```python
from build123d import *

# Parameters (mm, degrees)
SKETCH1_R           = 11
SKETCH1_R_2         = 5.375
SKETCH1_R_3         = 1.475
BOSS_EXTRUDE1_DEPTH = 3
SKETCH6_R           = 1.475
CUT_EXTRUDE1_DEPTH  = 11


with BuildPart() as part:
    # Sketch1 → Boss-Extrude1 (new body)
    with BuildSketch(Plane(origin=(0, 0, 0), x_dir=(1, 0, 0), z_dir=(0, 1, 0))):
        with Locations(Location((0, 0, 0), (0, 0, 270))):
            Circle(SKETCH1_R)
        with Locations(Location((0, 0, 0), (0, 0, 270))):
            Circle(SKETCH1_R_2, mode=Mode.SUBTRACT)
        with Locations(Location((-5.657708628, -5.655999742, 0), (0, 0, 270))):
            Circle(SKETCH1_R_3, mode=Mode.SUBTRACT)
        with Locations(Location((-5.657708628, 5.655999742, 0), (0, 0, 270))):
            Circle(SKETCH1_R_3, mode=Mode.SUBTRACT)
        with Locations(Location((5.657708628, 5.655999742, 0), (0, 0, 270))):
            Circle(SKETCH1_R_3, mode=Mode.SUBTRACT)
        with Locations(Location((5.657708628, -5.655999742, 0), (0, 0, 270))):
            Circle(SKETCH1_R_3, mode=Mode.SUBTRACT)
    extrude(amount=BOSS_EXTRUDE1_DEPTH)

    # Sketch5 → Revolve1 (revolve)
    with BuildSketch(Plane(origin=(0, 0, 0), x_dir=(0, 0, -1), z_dir=(1, 0, 0))):
        Polygon((5.375, 4.5), (5.375, 3), (11, 3), align=None)
    revolve(axis=Axis((0, 0, 0), (0, 1, 0)))

    # Sketch6 → Cut-Extrude1 (cut)
    with BuildSketch(Plane.XZ):
        with Locations(Location((-5.657708628, 5.655999742, 0), (0, 0, 221.262911431))):
            Circle(SKETCH6_R)
        with Locations(Location((-5.657708628, -5.655999742, 0), (0, 0, 224.999958606))):
            Circle(SKETCH6_R)
        with Locations(Location((5.657708628, 5.655999742, 0), (0, 0, 225.00013267))):
            Circle(SKETCH6_R)
        with Locations(Location((5.657708628, -5.655999742, 0), (0, 0, 228.738417152))):
            Circle(SKETCH6_R)
    extrude(amount=-CUT_EXTRUDE1_DEPTH, mode=Mode.SUBTRACT)


solid = part.part
```
The listing builds one solid part. Answer for the finished solid, in the listing's coordinates (mm). Round coordinates to 2 decimals unless told otherwise and drop trailing zeros. Loops run counter-clockwise (first coordinate to the right, second up) from the corner with the lowest first, then second, coordinate; pieces in that order, holes last.
Q1. Find the intervals of material crossed by line 1 (Z direction, x = 6.5, y = 0.3); line 2 (X direction, y = 2.25, z = -6.75); line 3 (X direction, y = 1.35, z = 6.25), in increasing order.
Q2. Section B-B, the plane z = 0 is taken. Determine the outline of the cut face in (x, y) (3 decimals), then the cut area to 3 significant figures.
Q3. Section C-C, the plane z = 6 is taken. Count the separate pieces of the cut face and the enclosed holes in it, then the cut area to 3 significant figures.
Q4. Section A-A, the plane x = 0 is taken. Determine the outline of the cut face in (y, z) (3 decimals).
Q5. Given pin 1 Ø2 at (x, y) = (-3, 3.5) entering from +Z; pin 2 Ø2 at (x, z) = (6, -7.5) entering from +Y, each flat-ended and moving along its own axis, determine where each tip first touches the part or whether it passes through.
Completed:
1. line 1: z = -8.87 to -6.87, -4.45 to 4.45, 6.87 to 8.87
1. line 2: x = -8.69 to -6.65, -4.67 to 4.67, 6.65 to 8.69
1. line 3: x = -9.05 to -7.01, -4.31 to 4.31, 7.01 to 9.05
2. outline: (-11, 0) - (-5.375, 0) - (-5.375, 4.5) - (-11, 3) - close; (5.375, 0) - (11, 0) - (11, 3) - (5.375, 4.5) - close
2. area: 42.2 mm2
3. separate pieces: 3
3. enclosed holes: 0
3. area: 49.3 mm2
4. outline: (0, -11) - (3, -11) - (4.5, -5.375) - (0, -5.375) - close; (0, 5.375) - (4.5, 5.375) - (3, 11) - (0, 11) - close
5. pin 1: stops at z = 10.79
5. pin 2: stops at y = 3.61
